The listing builds one solid part. Answer for the finished solid, in the listing's coordinates (mm). A direction names the side the tool comes from. Round coordinates to 2 decimals unless told otherwise and drop trailing zeros. Write each loop counter-clockwise with the first axis right and the second up, starting at its lowest first coordinate (ties: lowest second). Pieces come first, ordered by that corner, then holes.
Item 1: Find the intervals of material crossed by probe 1 along X at (y, z) = (5.25, 0.65) (3 decimals); probe 2 along Z at (x, y) = (-0.5, 4.5); probe 3 along X at (y, z) = (5.75, 2.2) (3 decimals), in increasing order.
Item 2: This flat-tipped pin is pushed along its axis until it touches: pin 1 (1.5 mm diameter, centred on x = -2, z = 1.5, fed in from -Y). Where does it stop, or does it pass through?
Item 3: Find section B-B on x = -1.75. Give the vertices of the cut face in (y, z).
Item 4: A tool of negligible diameter and unlimited length cuts with its end or side. For faces 5 (the face through (3.58, -0.86, 0.12)), 6 (the face through (-3.175, -1, -1)), 7 (the face through (-1, 3, 1.95)), from which of +Z, -Z, +X, -X, +Y, -Y can it reach the whole face along a straight path? Write none if from no direction.
Item 5: Find section C-C on z = -2.35. Give the vertices of the cut face in (x, y) (3 decimals).
Item 6: For a pull along Z with two mould halves and no side action, classify faces 1 (the face through (0, 3, 2.8)), 2 (the face through (-2.375, 3, 0)), 3 (the face through (0, 3, -2.8)), 4 (the face through (3.6, -1.75, -1.7)) as +Z half, -Z half, draft (parallel to the pull), parting line (faces both ways), or undercut.
Item 7: Find section A-A on y = 1.5. Give the vertices of the cut face in (x, z) (3 decimals), then the cut area to 3 significant figures.
Item 8: Find section D-D on y = -1. Give the vertices of the cut face in (x, z) (3 decimals).
```python
from build123d import *

# Parameters (mm, degrees)
F0_W     = 1.6
F0_H     = 0.85
F0_H_2   = 0.7
F1_DEPTH = 6
F0_W_2   = 0.4
F0_H_3   = 0.4
F2_DEPTH = 0.1
F4_DEPTH = 0.8
F6_DEPTH = 0.8


with BuildPart() as f1:
    # F0 (on Front) → F1 (new body)
    with BuildSketch(Plane.XZ):
        Polygon((-2.375, 1.95), (-3.975, 1.95), (-3.975, -2.8), (2.375, -2.8), (2.375, -2.1), (-2.375, -2.1), align=None)
        with Locations((-3.175, 2.375)):
            Rectangle(F0_W, F0_H)
        Polygon((3.975, 2.8), (-2.375, 2.8), (-2.375, 1.95), (-0.4, 1.95), (-0.4, 2.35), (0, 2.35), (0.4, 2.35), (0.4, 1.95), (2.375, 1.95), (2.375, -2.1), (3.975, -2.1), align=None)
        with Locations((3.175, -2.45)):
            Rectangle(F0_W, F0_H_2)
    extrude(amount=-F1_DEPTH)

    # F0 (on Front) → F2 (join)
    with BuildSketch(Plane.XZ):
        Polygon((-0.4, 1.95), (-2.375, 1.95), (-2.375, -2.1), (2.375, -2.1), (2.375, 1.95), (0.4, 1.95), (0, 1.95), align=None)
        with Locations((-0.2, 2.15)):
            Rectangle(F0_W_2, F0_H_3)
        with Locations((0.2, 2.15)):
            Rectangle(F0_W_2, F0_H_3)
    extrude(amount=-F2_DEPTH)

    # F3 (on face) → F4 (join)
    with BuildSketch(Plane.YZ.offset(3.975)):
        Polygon((0, -2.8), (0, 0.8), (-1.75, -0.582549), (-1.75, -2.8), align=None)
    extrude(amount=-F4_DEPTH)

    # F5 (on face) → F6 (join)
    with BuildSketch(Plane(origin=(-3.975, 0, 0), x_dir=(0, -1, 0), z_dir=(-1, 0, 0))):
        Polygon((1.75, -0.582549), (0, 0.8), (0, -2.8), (1.75, -2.8), align=None)
    extrude(amount=-F6_DEPTH)


solid = f1.part
```
Check values:
1. probe 1: x = -3.975 to -2.375, 2.375 to 3.975
1. probe 2: z = -2.8 to -2.1, 1.95 to 2.8
1. probe 3: x = -3.975 to -0.4, 0.4 to 3.975
2. pin 1: stops at y = 0
3. outline: (0, -2.8) - (6, -2.8) - (6, -2.1) - (0.1, -2.1) - (0.1, 1.95) - (6, 1.95) - (6, 2.8) - (0, 2.8) - close
4. face 5: +Z, +X, -X, -Y
4. face 6: +Z, -Z, -Y
4. face 7: +Y
5. outline: (-3.975, -1.75) - (-3.175, -1.75) - (-3.175, 0) - (3.175, 0) - (3.175, -1.75) - (3.975, -1.75) - (3.975, 6) - (-3.975, 6) - close
6. face 1: +Z half
6. face 2: undercut
6. face 3: -Z half
6. face 4: draft
7. outline: (-3.975, -2.8) - (3.975, -2.8) - (3.975, 2.8) - (-3.975, 2.8) - close; hole (-2.375, -2.1) - (2.375, -2.1) - (2.375, 1.95) - (0.4, 1.95) - (0.4, 2.35) - (-0.4, 2.35) - (-0.4, 1.95) - (-2.375, 1.95) - close
7. area: 25.0 mm2
8. outline: (-3.975, -2.8) - (-3.175, -2.8) - (-3.175, 0.01) - (-3.975, 0.01) - close; (3.175, -2.8) - (3.975, -2.8) - (3.975, 0.01) - (3.175, 0.01) - close
